CAD build for the part. Positions are in the model's coordinates, mm. A direction names the side the tool comes from. Coordinates: 2 decimals unless noted, no trailing zeros. Write each loop counter-clockwise with the first axis right and the second up, starting at its lowest first coordinate (ties: lowest second). Pieces come first, ordered by that corner, then holes.
```python
from build123d import *

# Parameters (mm, degrees)
BOSS_EXTRUDE1_DEPTH = 194.633333333
FILLET1_R           = 0.6
FILLET2_R           = 0.2


with BuildPart() as part:
    # Sketch1 → Boss-Extrude1 (new body)
    with BuildSketch(Plane.XY):
        Polygon((-5.7, 3.9), (5.7, 3.9), (5.7, 2.4), (4.9, 2.4), (4.9, -2.4), (-4.9, -2.4), (-4.9, 2.4), (-5.7, 2.4), align=None)
    extrude(amount=BOSS_EXTRUDE1_DEPTH)

    # Fillet1
    fillet1_edges = [part.edges().sort_by_distance(p)[0] for p in [
        (-4.9, 2.4, 97.316666667),
        (4.9, 2.4, 97.316666667),
    ]]
    fillet(fillet1_edges, radius=FILLET1_R)

    # Fillet2
    fillet2_edges = [part.edges().sort_by_distance(p)[0] for p in [
        (-5.7, 2.4, 97.316666667),
        (5.7, 2.4, 97.316666667),
    ]]
    fillet(fillet2_edges, radius=FILLET2_R - 0.0001)  # a hair under: the kernel refuses the full size


solid = part.part
```
Item 1: Flat gauge pins, fed straight in: pin 1 Ø2 at (y, z) = (0.5, 110.5) entering from -X; pin 2 Ø2 at (y, z) = (0.5, 158) entering from +X. Where does each tip first touch, or does it go through?
Item 2: Saw through at B-B, the plane y = -0.75. Write the cut outline in (x, z).
Item 3: Which spindle directions (+Z, -Z, +X, -X, +Y, -Y) get a long thin tool onto all of the face, cutting with end or side? Do faces 1 (the flat face through (0, -2.4, 96)), 2 (the flat face through (-4.9, 0, 96)), 3 (the flat face through (4.9, 0, 96)). Say none if no direction does.
Item 4: Wall check: line 1 along X through (y, z) = (-0.5, 126.5). Give the ranges that are in metal, low to high.
Working result:
1. pin 1: stops at x = -4.9
1. pin 2: stops at x = 4.9
2. outline: (-4.9, 0) - (4.9, 0) - (4.9, 194.63) - (-4.9, 194.63) - close
3. face 1: +Z, -Z, +X, -X, -Y
3. face 2: +Z, -Z, -X, -Y
3. face 3: +Z, -Z, +X, -Y
4. line 1: x = -4.9 to 4.9
